Part model, mm, in its own coordinate system. A direction names the side the tool comes from. Give positions to 0.01 mm unless a question says otherwise; leave off trailing zeros. Loops run counter-clockwise (first coordinate to the right, second up) from the corner with the lowest first, then second, coordinate; pieces in that order, holes last. Notation, with made-up numbers: M 49,74.25 L 93,74.25 A26 ccw 93,95.25 Z; hole C -20.5,31 d8. An arc over 180 degrees is marked long. Answer in a Markdown table with one row per item.
from build123d import *

# Parameters (mm, degrees)
SKETCH_1_R          = 11.75
EXTRUDE_1_DEPTH     = 10
SKETCH_1_3_R        = 6
EXTRUDE_2_DEPTH     = 4
SKETCH_1_4_R        = 5
EXTRUDE_3_DEPTH     = 26
CHAMFER_1_SIZE      = 0.6
SKETCH_2_R          = 4
EXTRUDE_4_DEPTH     = 8
CHAMFER_2_SIZE      = 0.6
CUT_EXTRUDE_1_DEPTH = 10


with BuildPart() as part:
    # Sketch 1 → Extrude 1 (new body)
    with BuildSketch(Plane(origin=(0, 0, 0), x_dir=(1, 0, 0), z_dir=(0, 1, 0))):
        with Locations(Location((0, 0, 0), (0, 0, 270))):
            Circle(SKETCH_1_R)
    extrude(amount=EXTRUDE_1_DEPTH)

    # Sketch 1_3 → Extrude 2 (add)
    with BuildSketch(Plane(origin=(0, 0, 0), x_dir=(1, 0, 0), z_dir=(0, 1, 0))):
        with Locations(Location((0, 0, 0), (0, 0, 270))):
            Circle(SKETCH_1_3_R)
    extrude(amount=-EXTRUDE_2_DEPTH)

    # Sketch 1_4 → Extrude 3 (add)
    with BuildSketch(Plane(origin=(0, 0, 0), x_dir=(1, 0, 0), z_dir=(0, 1, 0))):
        with Locations(Location((0, 0, 0), (0, 0, 270))):
            Circle(SKETCH_1_4_R)
    extrude(amount=-EXTRUDE_3_DEPTH)

    # Chamfer 1
    chamfer_1_edges = [part.edges().sort_by_distance(p)[0] for p in [
        (0, -26, -5),
    ]]
    chamfer(chamfer_1_edges, length=CHAMFER_1_SIZE)

    # Sketch 2 → Extrude 4 (add)
    with BuildSketch(Plane(origin=(0, 10, 0), x_dir=(1, 0, 0), z_dir=(0, 1, 0))):
        with Locations(Location((0, 0, 0), (0, 0, 270))):
            Circle(SKETCH_2_R)
    extrude(amount=EXTRUDE_4_DEPTH)

    # Chamfer 2
    chamfer_2_edges = [part.edges().sort_by_distance(p)[0] for p in [
        (0, 18, -4),
    ]]
    chamfer(chamfer_2_edges, length=CHAMFER_2_SIZE)

    # Sketch 3 → Cut-Extrude 1 (cut)
    with BuildSketch(Plane(origin=(-3.5, 0, 0), x_dir=(0, 0, -1), z_dir=(1, 0, 0))):
        with BuildLine():
            Line((-2, -22.2), (-2, -7.2))
            ThreePointArc((-2, -7.2), (0, -5.2), (2, -7.2))
            Line((2, -7.2), (2, -22.2))
            ThreePointArc((2, -22.2), (0, -24.2), (-2, -22.2))
        make_face()
    extrude(amount=-CUT_EXTRUDE_1_DEPTH, mode=Mode.SUBTRACT)


solid = part.part
(1) Saw through at A-A (z = 0). Write the cut outline in (x, y).
Recorded:
| item | result |
|---|---|
| outline | M -11.75,0 L -6,0 L -6,-4 L -5,-4 L -5,-5.2 L -3.5,-5.2 L -3.5,-24.2 L -5,-24.2 L -5,-25.4 L -4.4,-26 L 4.4,-26 L 5,-25.4 L 5,-4 L 6,-4 L 6,0 L 11.75,0 L 11.75,10 L 4,10 L 4,17.4 L 3.4,18 L -3.4,18 L -4,17.4 L -4,10 L -11.75,10 Z |
(2) Saw through at B-B (x = 0). Write the cut outline in (y, z).
Recorded:
| item | result |
|---|---|
| outline | M -26,-4.4 L -25.4,-5 L -4,-5 L -4,-6 L 0,-6 L 0,-11.75 L 10,-11.75 L 10,-4 L 17.4,-4 L 18,-3.4 L 18,3.4 L 17.4,4 L 10,4 L 10,11.75 L 0,11.75 L 0,6 L -4,6 L -4,5 L -25.4,5 L -26,4.4 Z |
(3) Saw through at C-C (y = -12). Write the cut outline in (x, z).
Recorded:
| item | result |
|---|---|
| outline | M -4.58,-2 A5 ccw long -4.58,2 L -3.5,2 L -3.5,-2 Z |
(4) Pin check, flat tips, straight feed: pin 1 Ø1.5 at (x, z) = (-7.5, -6.5) entering from -Y; pin 2 Ø4.5 at (y, z) = (-13.5, 1) entering from -X; pin 3 Ø5 at (x, y) = (-5, -6.5) entering from +Z; pin 4 Ø12 at (x, z) = (-5.5, 1) entering from +Y. Stop position of each tip, or through.
Recorded:
| item | result |
|---|---|
| pin 1 | stops at y = 0 |
| pin 2 | stops at x = -4.58 |
| pin 3 | stops at z = 4.33 |
| pin 4 | stops at y = 18 |
(5) Which spindle directions (+Z, -Z, +X, -X, +Y, -Y) get a long thin tool onto all of the face, cutting with end or side? Do faces 1 (the face through (4, -15, 3)), 2 (the face through (-3.905, 13.648, -0.867)), 3 (the face through (0, -26, 0)), 4 (the face through (-4.1, -5.2, 0)), 5 (the face through (7.9, 4.9, -8.7)). Say none if no direction does.
Recorded:
| item | result |
|---|---|
| face 1 | -Y |
| face 2 | +Y |
| face 3 | +Z, -Z, +X, -X, -Y |
| face 4 | -X |
| face 5 | +Y, -Y |
(6) Drill centre lines: line 1 along Y through (x, z) = (-0.5, -10.5); line 2 along X through (y, z) = (9, -6.5); line 3 along Z through (x, y) = (-2.5, 13). Where is each one in solid material? Low to high.
Recorded:
| item | result |
|---|---|
| line 1 | y = 0 to 10 |
| line 2 | x = -9.79 to 9.79 |
| line 3 | z = -3.12 to 3.12 |
(7) Pull direction Y, two halves, no side cores. Call faces 6 (the face through (-4.1, -24.2, 0)), 7 (the face through (0, 18, 0)), 8 (the face through (-5, 0, 5)): +Y half, -Y half, draft (parallel to the pull), parting line (faces both ways), or undercut.
Recorded:
| item | result |
|---|---|
| face 6 | undercut |
| face 7 | +Y half |
| face 8 | -Y half |
(8) Saw through at D-D (y = 12). Write the cut outline in (x, z).
Recorded:
| item | result |
|---|---|
| outline | C 0,0 d8 |
